from build123d import *

# Parameters (mm, degrees)
ESQUISSE1_W             = 59
ESQUISSE1_H             = 59
BOSS_EXTRU_1_DEPTH      = 70
ENL_V_MAT_EXTRU_1_REACH = 61
ESQUISSE2_R             = 2
ESQUISSE3_R             = 11
ENL_V_MAT_EXTRU_2_DEPTH = 25
ENL_V_MAT_EXTRU_3_REACH = 61
ESQUISSE4_R             = 5


with BuildPart() as part:
    # Esquisse1 → Boss.-Extru.1 (new body)
    with BuildSketch(Plane(origin=(0, 0, 0), x_dir=(1, 0, 0), z_dir=(0, 1, 0))):
        with Locations((0.20896915, -12.058522539)):
            Rectangle(ESQUISSE1_W, ESQUISSE1_H)
    extrude(amount=BOSS_EXTRU_1_DEPTH)

    # Esquisse2 → Enlèv. mat.-Extru.1 (cut, up to next)
    with BuildSketch(Plane.XY.offset(41.558522539), mode=Mode.PRIVATE) as enl_v_mat_extru_1_sk1:
        with Locations((-15.29103085, 14)):
            Circle(ESQUISSE2_R)
    enl_v_mat_extru_1_tool1 = extrude(enl_v_mat_extru_1_sk1.sketch, amount=-ENL_V_MAT_EXTRU_1_REACH, mode=Mode.PRIVATE) & part.part
    add(enl_v_mat_extru_1_tool1.solids().sort_by_distance((-15.291031, 14, 41.558523))[0], mode=Mode.SUBTRACT)
    # Esquisse2 → Enlèv. mat.-Extru.1 (cut, up to next)
    with BuildSketch(Plane.XY.offset(41.558522539), mode=Mode.PRIVATE) as enl_v_mat_extru_1_sk2:
        with Locations((15.70896915, 14)):
            Circle(ESQUISSE2_R)
    enl_v_mat_extru_1_tool2 = extrude(enl_v_mat_extru_1_sk2.sketch, amount=-ENL_V_MAT_EXTRU_1_REACH, mode=Mode.PRIVATE) & part.part
    add(enl_v_mat_extru_1_tool2.solids().sort_by_distance((15.708969, 14, 41.558523))[0], mode=Mode.SUBTRACT)

    # Esquisse3 → Enlèv. mat.-Extru.2 (cut)
    with BuildSketch(Plane(origin=(0, 70, 0), x_dir=(1, 0, 0), z_dir=(0, 1, 0))):
        with Locations((11.70896915, -12.058522539)):
            Circle(ESQUISSE3_R)
    extrude(amount=-ENL_V_MAT_EXTRU_2_DEPTH, mode=Mode.SUBTRACT)

    # Esquisse4 → Enlèv. mat.-Extru.3 (cut, up to next)
    with BuildSketch(Plane(origin=(29.70896915, 0, 0), x_dir=(0, 0, -1), z_dir=(1, 0, 0)), mode=Mode.PRIVATE) as enl_v_mat_extru_3_sk1:
        with Locations((-12.058522539, 50)):
            Circle(ESQUISSE4_R)
    enl_v_mat_extru_3_tool1 = extrude(enl_v_mat_extru_3_sk1.sketch, amount=-ENL_V_MAT_EXTRU_3_REACH, mode=Mode.PRIVATE) & part.part
    add(enl_v_mat_extru_3_tool1.solids().sort_by_distance((29.708969, 50, 12.058523))[0], mode=Mode.SUBTRACT)


solid = part.part
The listing builds one solid part. Answer for the finished solid, in the listing's coordinates (mm). A direction names the side the tool comes from. Give positions to 0.01 mm unless a question says otherwise; leave off trailing zeros. Write each loop counter-clockwise with the first axis right and the second up, starting at its lowest first coordinate (ties: lowest second). Pieces come first, ordered by that corner, then holes.
Item 1: Which of the six approach directions +Z, -Z, +X, -X, +Y, -Y give full straight-line access (tool end or side, diameter ignored) to faces 4 (the flat face through (0, 35, 41.559)), 5 (the cylindrical face through (25.67, 45.12, 13.14)), 6 (the cylindrical face through (0.72, 57.68, 11.57))?
Item 2: A flat-ended cylindrical pin translates along its axis: P1, Ø17.5, axis at x = 11.71, z = 12.06, coming from the +Y side. Find the tip coordinate at first contact, or state that the pin passes through.
Item 3: Section B-B, the plane y = 14 is taken. Write down the section's boundary in (x, z).
Item 4: Section D-D, the plane x = -15.5 is taken. Write down the section's boundary in (y, z).
Item 5: Find the intervals of material crossed by line 1 along Z through (x, y) = (18.5, 51); line 2 along Z through (x, y) = (5, 61.5); line 3 along Y through (x, z) = (7, 6), in increasing order.
Item 6: Section C-C, the plane y = 50 is taken. Write down the section's boundary in (x, z).
Item 7: Determine the mould class of faces 1 (the flat face through (0, 0, 12)), 2 (the cylindrical face through (14.235, 15.352, 12.472)), 3 (the flat face through (0, 70, 12)) for opening direction Y: released by +Y, released by -Y, zero draft, split by the parting line, or undercut.
Item 8: Section A-A, the plane z = 9 is taken. Write down the section's boundary in (x, y), plus the area to 3 significant figures.
Completed:
1. face 4: +Z, +X, -X, +Y, -Y
1. face 5: +X
1. face 6: +Y
2. P1: stops at y = 45
3. outline: (-29.29, -17.44) - (-17.29, -17.44) - (-17.29, 41.56) - (-29.29, 41.56) - close; (-13.29, -17.44) - (13.71, -17.44) - (13.71, 41.56) - (-13.29, 41.56) - close; (17.71, -17.44) - (29.71, -17.44) - (29.71, 41.56) - (17.71, 41.56) - close
4. outline: (0, -17.44) - (12.01, -17.44) - (12.01, 41.56) - (0, 41.56) - close; (15.99, -17.44) - (70, -17.44) - (70, 41.56) - (15.99, 41.56) - close
5. line 1: z = -17.44 to 3.41, 20.71 to 41.56
5. line 2: z = -17.44 to 3.34, 20.78 to 41.56
5. line 3: y = 0 to 45
6. outline: (-29.29, -17.44) - (29.71, -17.44) - (29.71, 7.06) - (21.51, 7.06) arc R11 cw (long way) to (21.51, 17.06) - (29.71, 17.06) - (29.71, 41.56) - (-29.29, 41.56) - close
7. face 1: released by -Y
7. face 2: undercut
7. face 3: released by +Y
8. outline: (-29.29, 0) - (29.71, 0) - (29.71, 46.04) - (22.28, 46.04) - (22.28, 45) - (1.14, 45) - (1.14, 70) - (-29.29, 70) - close; (22.28, 53.96) - (29.71, 53.96) - (29.71, 70) - (22.28, 70) - close; hole circle Ø4 at (-15.29, 14); hole circle Ø4 at (15.71, 14)
8. area: 3,520 mm2
